Build history of the part. All positions in model axes, mm. A direction names the side the tool comes from. Give positions to 0.01 mm unless a question says otherwise; leave off trailing zeros. Order: outer loops, then holes, each group sorted by start corner. A loop starts at its lowest first (then second) coordinate and runs counter-clockwise, first axis right, second up. Notation, with made-up numbers: (-16, 31.5) -> (20, 31.5) arc R23 ccw to (20, 63.5) -> close; hole circle Ø4 at (-11, 68.5). An arc over 180 degrees is marked (long way). Write item = value, one per line. Start each with the question number.
Autodesk Inventor part; units mm, degrees
ref_plane "YZ Plane" through (0, 0, 0) normal (1, 0, 0) x (0, 1, 0)
ref_plane "XZ Plane" through (0, 0, 0) normal (0, 1, 0) x (-1, 0, 0)
ref_plane "XY Plane" through (0, 0, 0) normal (0, 0, 1) x (1, 0, 0)
sketch "Sketch1" plane through (0, 0, 0) normal (0, 1, 0) x (-1, 0, 0)
  line L0 (0, 0) -> (10, 0)
  line L1 (10, 0) -> (10, -28)
  line L2 (10, -28) -> (0, -28)
  line L3 (0, -28) -> (0, 0)
extrude "Extrusion1" add sketch "Sketch1" along normal blind 20
sketch "Sketch6" plane through (0, 0, 0) normal (1, 0, 0) x (0, 0, -1)
  point P0 (0, 0)
sketch "Sketch7" plane through (0, 0, 0) normal (1, 0, 0) x (0, 0, -1)
  circle A0 centre (14, 5) radius 2.25
  point P0 (0, 0)
  dimension "d14" = 4.5
extrude "Extrusion6" cut sketch "Sketch7" against normal blind 2.5
sketch "Sketch8" plane through (0, 0, 0) normal (1, 0, 0) x (0, 0, -1)
  line L0 (0, 0) -> (0, 20)
  line L1 (0, 0) -> (-0.5, 0)
  line L2 (-0.5, 0) -> (-0.5, 20)
  line L3 (-0.5, 20) -> (0, 20)
  line L4 (0, 20) -> (0, 0)
  line L5 (28, 0) -> (28.5, 0)
  line L6 (28.5, 0) -> (28.5, 20)
  line L7 (28.5, 20) -> (28, 20)
  line L8 (28, 20) -> (28, 0)
  dimension "d17" = 0.5
  dimension "d18" = 0.5
extrude "Extrusion7" add sketch "Sketch8" against normal blind 10
properties part number "Kolv"
(1) Wall check: line 1 (Y direction, x = -1, z = -14); line 2 (Y direction, x = -1.75, z = -15.25); line 3 (X direction, y = 5, z = -14.75). Give the ranges that are in metal, low to high. Write a range as [from, to].
(2) Flat gauge pin, fed straight in: P1, Ø1.3, axis at y = 4, z = -13.5, coming from the +X side. Where does the tip first touch, or does it go through?
(3) Mould opens along Y. For faces 1 (the face through (-5, 10, 0.5)), 2 (the face through (-5, 20, -14)), 3 (the face through (-2.5, 5, -14)) say: released by +Y, released by -Y, zero draft, split by the parting line, or undercut.
(4) Cut at A-A, the plane z = -14. Give the cut face in (x, y).
(5) Cut at C-C, the plane y = 5. Give the cut face in (x, z).
(6) Cut at B-B, the plane x = -1.25. Give the cut face in (y, z), plus the area to 3 significant figures.
(7) 3-axis set-ups, long thin cutter, end or side, ignore diameter. For faces 4 (the face through (-1.232, 5.676, -16.146)), 5 (the face through (-10, 10, -14)): which of +Z, -Z, +X, -X, +Y, -Y reach the whole face in a straight line?
Results:
q1.line_1 = [0, 2.75], [7.25, 20]
q1.line_2 = [0, 3.13], [6.87, 20]
q1.line_3 = [-10, -2.5]
q2.P1 = -2.5
q3.face_1 = zero draft
q3.face_2 = released by +Y
q3.face_3 = undercut
q4.outline = (-10, 0) -> (0, 0) -> (0, 2.75) -> (-2.5, 2.75) -> (-2.5, 7.25) -> (0, 7.25) -> (0, 20) -> (-10, 20) -> close
q5.outline = (-10, -28.5) -> (0, -28.5) -> (0, -16.25) -> (-2.5, -16.25) -> (-2.5, -11.75) -> (0, -11.75) -> (0, 0.5) -> (-10, 0.5) -> close
q6.outline = (0, -28.5) -> (20, -28.5) -> (20, 0.5) -> (0, 0.5) -> close; hole circle Ø4.5 at (5, -14)
q6.area = 564 mm2
q7.face_4 = +X
q7.face_5 = +Z, -Z, -X, +Y, -Y
